Input: part model. Units: mm. Frame: model coordinates. A direction names the side the tool comes from. Coordinates: 2 decimals unless noted, no trailing zeros. Loops run counter-clockwise (first coordinate to the right, second up) from the corner with the lowest first, then second, coordinate; pieces in that order, holes last. Notation, with made-up numbers: (-15, -32.75) - (6, -32.75) arc R24 ccw to (6, -6.75) - close; hole circle Ø4 at (5, 58). An arc over 180 degrees is marked (long way). Use one line per item in the form item = value.
from build123d import *

# Parameters (mm, degrees)
F0_W      = 28.5392315894
F0_H      = 48.2956362042
F1_DEPTH  = 25.4
F1_FACE_W = 28.5392315894
F1_FACE_H = 48.2956362042
F2_ANGLE  = 90
F3_DEPTH  = 38.1
F4_W      = 26.9696157947
F4_H      = 26.9696157947
F5_DEPTH  = 50.14334
F6_W      = 26.9748
F6_H      = 6.35
F7_DEPTH  = 25.4
F9_DEPTH  = 38.1
F11_DEPTH = 12.7


with BuildPart() as f1:
    # F0 (on Front) → F1 (new body)
    with BuildSketch(Plane.XZ):
        with Locations((-3.175, -0.3527777778)):
            Rectangle(F0_W, F0_H)
        Polygon((-12.7, -19.4027777778), (-12.7, 18.6972222222), (6.35, 18.6972222222), (6.35, 2.8222222222), (-1.27, 2.8222222222), (-1.27, -3.5277777778), (6.35, -3.5277777778), (6.35, -19.4027777778), align=None, mode=Mode.SUBTRACT)
    extrude(amount=F1_DEPTH)

    # F1_face (on face) → F2 (revolve)
    with BuildSketch(Plane(origin=(-2.7804632911, -25.4, -0.3527777778), x_dir=(1, 0, 0), z_dir=(0, -1, 0))):
        with Locations((-0.3945367089, 0)):
            Rectangle(F1_FACE_W, F1_FACE_H)
        Polygon((9.1304632911, -19.05), (-9.9195367089, -19.05), (-9.9195367089, 19.05), (9.1304632911, 19.05), (9.1304632911, 3.175), (1.5104632911, 3.175), (1.5104632911, -3.175), (9.1304632911, -3.175), align=None, mode=Mode.SUBTRACT)
    revolve(axis=Axis((11.0946157947, -25.4, -0.3527777778), (0, 0, 1)), revolution_arc=F2_ANGLE)

    # F3 (add): a face of the model
    f3_faces = [f1.faces().sort_by_distance(p)[0] for p in [
        (11.0946157947, -22.3630131274, -0.3527777778),
    ]]
    extrude(f3_faces, amount=F3_DEPTH)

    # F4 (on face) → F5 (cut, symmetric)
    with BuildSketch(Plane(origin=(0, 0, -24.5005958799), x_dir=(1, 0, 0), z_dir=(0, 0, -1))):
        with Locations((35.7098078974, 13.4848078974)):
            Rectangle(F4_W, F4_H)
    extrude(amount=F5_DEPTH, both=True, mode=Mode.SUBTRACT)

    # F6 (on face) → F7 (join)
    with BuildSketch(Plane(origin=(0, 0, -24.5005958799), x_dir=(1, 0, 0), z_dir=(0, 0, -1))):
        Polygon((22.2198247534, 33.3196136858), (22.225, 26.9696157947), (49.1946157947, 26.9915960246), (49.1946157947, 33.3415981335), align=None)
        with Locations((35.7072157947, 50.7642315894)):
            Rectangle(F6_W, F6_H)
        with BuildLine():
            Line((22.225, 0), (22.225, 26.9696157947))
            Line((22.225, 26.9696157947), (22.2198247534, 33.3196136858))
            Line((22.2198247534, 33.3196136858), (49.1946157947, 33.3415981335))
            Line((49.1946157947, 33.3415981335), (49.1946157947, 47.5892315894))
            Line((49.1946157947, 47.5892315894), (22.2198157947, 47.5892315894))
            Line((22.2198157947, 47.5892315894), (22.2198157947, 53.9392315894))
            Line((22.2198157947, 53.9392315894), (11.0946157947, 53.9392315894))
            ThreePointArc((11.0946157947, 53.9392315894), (-9.085668392, 45.5802841867), (-17.4446157947, 25.4))
            Line((-17.4446157947, 25.4), (-17.4446157947, 0))
            Line((-17.4446157947, 0), (22.225, 0))
        make_face()
    extrude(amount=F7_DEPTH)

    # F8 (on face) → F9 (cut)
    with BuildSketch(Plane.XZ.offset(53.9392315894)):
        with BuildLine():
            ThreePointArc((27.5649282947, -35.9276048839), (30.1446157947, -38.5072923839), (32.7243032947, -35.9276048839))
            Line((32.7243032947, -35.9276048839), (30.1446157947, -35.9276048839))
            Line((30.1446157947, -35.9276048839), (27.5649282947, -35.9276048839))
        make_face()
        with BuildLine():
            Line((30.1446157947, -35.9276048839), (32.7243032947, -35.9276048839))
            ThreePointArc((32.7243032947, -35.9276048839), (30.1446157947, -33.3479173839), (27.5649282947, -35.9276048839))
            Line((27.5649282947, -35.9276048839), (30.1446157947, -35.9276048839))
        make_face()
    extrude(amount=-F9_DEPTH, mode=Mode.SUBTRACT)

    # F11 (cut): a face of the model
    f11_faces = [f1.faces().sort_by_distance(p)[0] for p in [
        (22.225, -13.4848078974, -13.0527777778),
    ]]
    extrude(f11_faces, amount=-F11_DEPTH, mode=Mode.SUBTRACT)


solid = f1.part
Q1. Ray query, line 1 along Z through (x, y) = (30, -35); line 2 along Y through (x, z) = (12, 9); line 3 along Z through (x, y) = (4.5, -44.5). Return the intervals inside material, ascending. Write a range as [from, to].
Check values:
line_1 = [-49.9, -38.5], [-33.35, -19.4], [-3.53, 2.82], [18.7, 23.8]
line_2 = [-53.94, -49.19], [-30.14, -26.97]
line_3 = [-49.9, -19.4], [18.7, 23.8]
Q2. Cut plane A-A, the plane y = -15. Return loops of the section in (x, z) (3 decimals), then the cut area to 3 significant figures.
Check values:
outline = (-17.445, -49.901) - (9.525, -49.901) - (9.525, 23.795) - (-17.445, 23.795) - close; hole (-12.7, -19.403) - (6.35, -19.403) - (6.35, -3.528) - (-1.27, -3.528) - (-1.27, 2.822) - (6.35, 2.822) - (6.35, 18.697) - (-12.7, 18.697) - close
area = 1,310 mm²
Q3. Cut plane B-B, the plane z = 5. Return loops of the section in (x, y) (3 decimals), then the cut area to 3 significant figures.
Check values:
outline = (-17.445, -25.4) arc R28.539 ccw to (11.095, -53.939) - (49.195, -53.939) - (49.195, -49.195) - (11.095, -49.195) arc R23.795 cw to (-12.7, -25.4) - (-12.7, 0) - (-17.445, 0) - close; (6.35, -25.4) arc R4.745 ccw to (11.095, -30.145) - (49.195, -30.145) - (49.195, -26.97) - (9.525, -26.97) - (9.525, 0) - (6.35, 0) - close
area = 713 mm²
Q4. Cut plane D-D, the plane y = -32. Return loops of the section in (x, z).
Check values:
outline = (-16.67, -49.9) - (49.19, -49.9) - (49.19, -19.4) - (-11.77, -19.4) - (-11.77, 18.7) - (49.19, 18.7) - (49.19, 23.8) - (-16.67, 23.8) - close; (0.64, -3.53) - (49.19, -3.53) - (49.19, 2.82) - (0.64, 2.82) - close; hole circle Ø5.16 at (30.14, -35.93)
Q5. Pull-direction query (Z, two-part tool) for faces 1 (the flat face through (15, -33, -49.901)), 2 (the flat face through (-4, 0, -21)), 3 (the cylindrical face through (-5.915, -42.039, -0.086)); classes: pulls with the +Z half, pulls with the -Z half, needs draft (parallel to the pull), parting line crosses it, or undercut.
Check values:
face_1 = pulls with the -Z half
face_2 = needs draft
face_3 = undercut
Q6. Cut plane C-C, the plane x = 3.5. Return loops of the section in (y, z).
Check values:
outline = (-52.91, -49.9) - (0, -49.9) - (0, -19.4) - (-47.95, -19.4) - (-47.95, 18.7) - (0, 18.7) - (0, 23.8) - (-52.91, 23.8) - close; (-35.16, -3.53) - (0, -3.53) - (0, 2.82) - (-35.16, 2.82) - close
Q7. Set-up query: faces 4 (the flat face through (30, -49.195, -1)), 5 (the flat face through (9.525, -13, -13)), 6 (the flat face through (49.195, -40, -21)), 7 (the flat face through (11, -35, -19.403)), 8 (the flat face through (6.35, -13, 11)). Return all of +Z, -Z, +X, -X, +Y, -Y with unobstructed straight access to the full face (end or side cutting, diameter ignored); none if empty.
Check values:
face_4 = +X
face_5 = +Z, -Z, +X, +Y
face_6 = +Z, -Z, +X, +Y, -Y
face_7 = none
face_8 = +Y
Q8. First-contact query: P1, Ø3, axis at y = -42.5, z = -32, coming from the -X side; P2, Ø12.5, axis at y = -18.5, z = -3, coming from the +X side (3 decimals); P3, Ø19, axis at x = 36.5, z = -3.5, coming from the +Y side. Flat tips, straight axial feed; report the tip coordinate or a pass-through.
Check values:
P1 = -12.8
P2 = 9.525
P3 = -26.97
